Autodesk Fusion 360 part; units mm, degrees
sketch "Skizze1" plane through (0, 0, 0) normal (0, 0, 1) x (1, 0, 0)
  line L0 (0, 0) -> (125, 0)
  line L1 (125, 0) -> (125, 20)
  line L2 (125, 20) -> (0, 20)
  line L3 (0, 20) -> (0, 0)
  dimension "d1" = 125
  dimension "d2" = 20
extrude "Extrusion1" add sketch "Skizze1" along normal blind 10
sketch "Skizze2" plane through (0, 0, 10) normal (0, 0, 1) x (-1, 0, 0)
  line L0 (0, -20) -> (0, 0)
  line L1 (0, 0) -> (-125, 0)
  line L2 (-125, 0) -> (-125, -20)
  line L3 (-125, -20) -> (0, -20)
  circle A0 centre (-62.5, -10) radius 3.75
  dimension "d5" = 7.5
extrude "Extrusion2" cut sketch "Skizze2" against normal blind 10 contours A0
sketch "Skizze3" plane through (0, 0, 10) normal (0, 0, 1) x (-1, 0, 0)
  circle A0 centre (-62.5, -10) radius 3.75
  line L0 (0, -20) -> (0, 0)
  line L1 (0, 0) -> (-125, 0)
  line L2 (-125, 0) -> (-125, -20)
  line L3 (-125, -20) -> (0, -20)
  curve L4
  curve L5
  line L6 (-125, -10) -> (-119.5, -10)
  circle A1 centre (-5.5026, -10) radius 5
  circle A2 centre (-119.5, -10) radius 5
  dimension "d8" = 5.5
  dimension "d9" = 5.5
  dimension "d10" = 10
  dimension "d13" = 10
extrude "Extrusion4" add sketch "Skizze3" along normal blind 25 contours A2 | A1
extrude "Extrusion3" add sketch "Skizze3" along normal blind 10 contours A1
sketch "Skizze4" plane through (0, 0, 10) normal (0, 0, 1) x (1, 0, 0)
  circle A0 centre (62.5, 10) radius 3.8
  point P0 (62.5, 10)
  dimension "d16" = 7.6
extrude "Extrusion5" cut sketch "Skizze4" against normal blind 20
sketch "Skizze5" plane through (0, 0, 10) normal (0, 0, 1) x (1, 0, 0)
Read the model definition and answer for the solid it produces. Units are mm, in the model's axes. A direction names the side the tool comes from. Give positions to 0.01 mm unless a question says otherwise; leave off trailing zeros. Loops run counter-clockwise (first coordinate to the right, second up) from the corner with the lowest first, then second, coordinate; pieces in that order, holes last. Notation, with made-up numbers: (-11, 50) - (3, 50) arc R13 cw to (3, 72) - close; hole circle Ø5 at (0, 61). An arc over 180 degrees is marked (long way). Answer as CSV lines item,"result". Start each with the question number.
1) Find section D-D (z = 16). Write down the section's boundary in (x, y).
2) Straight lines are drawn through the part: L1, parallel to X at y = 10, z = 20; L2, parallel to Y at x = 62.5, z = 2; L3, parallel to Z at x = 50, y = 8. For each, find the intervals that lie inside material, in ascending order. Write a range as from..to.
3) Determine the mould class of faces 3 (the face through (0, 10, 5)), 4 (the face through (6.154, 14.957, 22.325)), 5 (the face through (120, 10, 35)) for opening direction X: released by +X, released by -X, zero draft, split by the parting line, or undercut.
4) Each of these flat-tipped pins is pushed along its axis until it touches: pin 1 Ø3 at (x, y) = (72.5, 7) entering from +Z; pin 2 Ø1 at (y, z) = (5, 24) entering from -X; pin 3 Ø8 at (y, z) = (9, 16) entering from -X; pin 4 Ø7 at (x, y) = (62.5, 10) entering from -Z. Where does it stop, or does it pass through?
5) Find section C-C (x = 119.5). Write down the section's boundary in (y, z).
6) Find section B-B (y = 10). Write down the section's boundary in (x, z), then the cut area to 3 significant figures.
7) Find section A-A (x = 62.5). Write down the section's boundary in (y, z).
8) Which of the six approach directions +Z, -Z, +X, -X, +Y, -Y give full straight-line access (tool end or side, diameter ignored) to faces 1 (the face through (125, 10, 5)), 2 (the face through (114.881, 8.085, 22.325))?
Findings below:
1,outline,"circle Ø10 at (5.5, 10); circle Ø10 at (119.5, 10)"
2,L1,"0.5..10.5, 114.5..124.5"
2,L2,"0..6.2, 13.8..20"
2,L3,"0..10"
3,face 3,"released by -X"
3,face 4,"undercut"
3,face 5,"zero draft"
4,pin 1,"z = 10"
4,pin 2,"x = 3.32"
4,pin 3,"x = 0.5"
4,pin 4,"through"
5,outline,"(0, 0) - (20, 0) - (20, 10) - (15, 10) - (15, 35) - (5, 35) - (5, 10) - (0, 10) - close"
6,outline,"(0, 0) - (58.7, 0) - (58.7, 10) - (10.5, 10) - (10.5, 35) - (0.5, 35) - (0.5, 10) - (0, 10) - close; (66.3, 0) - (125, 0) - (125, 10) - (124.5, 10) - (124.5, 35) - (114.5, 35) - (114.5, 10) - (66.3, 10) - close"
6,area,"1,670 mm^2"
7,outline,"(0, 0) - (6.2, 0) - (6.2, 10) - (0, 10) - close; (13.8, 0) - (20, 0) - (20, 10) - (13.8, 10) - close"
8,face 1,"+Z, -Z, +X, +Y, -Y"
8,face 2,"+Z"
